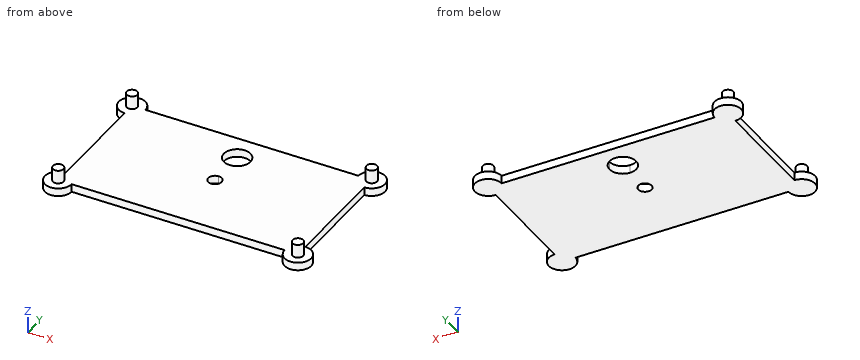
```python
from build123d import *

# Parameters (mm, degrees)
F0_R     = 2
F1_DEPTH = 3
F2_DEPTH = 8
F4_DEPTH = 4


with BuildPart() as f1:
    # F0 (on Top) → F1 (new body)
    with BuildSketch(Plane.XY):
        with BuildLine():
            Line((40, 25), (-40, 25))
            ThreePointArc((-40, 25), (-48.535534, 28.535534), (-45, 20))
            Line((-45, 20), (-45, -20))
            ThreePointArc((-45, -20), (-48.535534, -28.535534), (-40, -25))
            Line((-40, -25), (40, -25))
            ThreePointArc((40, -25), (48.535534, -28.535534), (45, -20))
            Line((45, -20), (45, 20))
            ThreePointArc((45, 20), (48.535534, 28.535534), (40, 25))
        make_face()
        with Locations((-45, -25)):
            Circle(F0_R, mode=Mode.SUBTRACT)
        with Locations((45, -25)):
            Circle(F0_R, mode=Mode.SUBTRACT)
        with Locations((-45, 25)):
            Circle(F0_R, mode=Mode.SUBTRACT)
        with Locations((45, 25)):
            Circle(F0_R, mode=Mode.SUBTRACT)
    extrude(amount=F1_DEPTH)

    # F0 (on Top) → F2 (join)
    with BuildSketch(Plane.XY):
        with Locations((-45, -25)):
            Circle(F0_R)
        with Locations((45, -25)):
            Circle(F0_R)
        with Locations((45, 25)):
            Circle(F0_R)
        with Locations((-45, 25)):
            Circle(F0_R)
    extrude(amount=F2_DEPTH)

    # F3 (on Top) → F4 (cut)
    with BuildSketch(Plane.XY):
        with BuildLine():
            ThreePointArc((2.5, 0), (1.767767, 1.767767), (0, 2.5))
            ThreePointArc((0, 2.5), (-1.767767, -1.767767), (2.5, 0))
        make_face()
        with BuildLine():
            ThreePointArc((5, 15), (-3.535534, 18.535534), (0, 10))
            ThreePointArc((0, 10), (3.535534, 11.464466), (5, 15))
        make_face()
    extrude(amount=F4_DEPTH, mode=Mode.SUBTRACT)


solid = f1.part
```
Part model, mm, in its own coordinate system. Round coordinates to 2 decimals unless told otherwise and drop trailing zeros. Order: outer loops, then holes, each group sorted by start corner. A loop starts at its lowest first (then second) coordinate and runs counter-clockwise, first axis right, second up. Notation, with made-up numbers: M 38,55.25 L 65,55.25 A26 cw 65,82.25 Z; hole C 19.25,11 d5. An arc over 180 degrees is marked long. Answer in a Markdown table with one row per item. Add a question column.
Q1. Wall check: L1, parallel to X at y = 15, z = 1.95; L2, parallel to X at y = 0, z = 1.7; L3, parallel to Y at x = 45, z = 4.5. Give the ranges that are in metal, low to high. Write a range as from..to.
Q2. Cut at C-C on x = 17.5. Give the cut face in (y, z), and give its area (3 significant figures).
Q3. Pin check, flat tips, straight feed: pin 1 (4 mm diameter, centred on y = 1, z = 3, fed in from +X); pin 2 (1.5 mm diameter, centred on x = -13.5, z = 1.5, fed in from +Y); pin 3 (3 mm diameter, centred on x = 13, y = 6.5, fed in from +Z); pin 4 (8 mm diameter, centred on x = 0, y = 15, fed in from -Z). Stop position of each tip, or through.
Q4. Cut at B-B on y = 9. Give the cut face in (x, z).
Q5. Cut at A-A on z = 4.75. Give the cut face in (x, y), and give its area (3 significant figures).
Established:
| question | item | result |
|---|---|---|
| 1 | L1 | x = -45..-5, 5..45 |
| 1 | L2 | x = -45..-2.5, 2.5..45 |
| 1 | L3 | y = -27..-23, 23..27 |
| 2 | outline | M -25,0 L 25,0 L 25,3 L -25,3 Z |
| 2 | area | 150 mm2 |
| 3 | pin 1 | stops at x = 45 |
| 3 | pin 2 | stops at y = 25 |
| 3 | pin 3 | stops at z = 3 |
| 3 | pin 4 | passes through |
| 4 | outline | M -45,0 L 45,0 L 45,3 L -45,3 Z |
| 5 | outline | C -45,-25 d4; C -45,25 d4; C 45,-25 d4; C 45,25 d4 |
| 5 | area | 50.3 mm2 |
